```python
from build123d import *

# Parameters (mm, degrees)
BOSS_EXTRUDE1_DEPTH = 0.9


with BuildPart() as part:
    # Sketch1 → Boss-Extrude1 (new body)
    with BuildSketch(Plane(origin=(0, 0, 0), x_dir=(1, 0, 0), z_dir=(0, 1, 0))):
        with BuildLine():
            Line((37, -29.25), (-37, -29.25))
            ThreePointArc((-37, -29.25), (-40.889087297, -27.639087297), (-42.5, -23.75))
            Line((-42.5, -23.75), (-42.5, 23.75))
            ThreePointArc((-42.5, 23.75), (-40.889087297, 27.639087297), (-37, 29.25))
            Line((-37, 29.25), (37, 29.25))
            ThreePointArc((37, 29.25), (40.889087297, 27.639087297), (42.5, 23.75))
            Line((42.5, 23.75), (42.5, -23.75))
            ThreePointArc((42.5, -23.75), (40.889087297, -27.639087297), (37, -29.25))
        make_face()
    extrude(amount=BOSS_EXTRUDE1_DEPTH)

    # Sweep1: sweep along a path in Sketch2
    with BuildLine(Plane(origin=(0, 0.9, 0), x_dir=(1, 0, 0), z_dir=(0, 1, 0))) as sweep1_path:
        Line((34.75, -21.75), (-34.75, -21.75))
        Line((-34.75, -21.75), (-34.75, 21.75))
        Line((-34.75, 21.75), (34.75, 21.75))
        Line((34.75, 21.75), (34.75, -21.75))
    # Sketch3 → Sweep1 (sweep)
    with BuildSketch(Plane.XY):
        with BuildLine():
            Line((-38.25, 0.9), (-31.25, 0.9))
            Line((-31.25, 0.9), (-31.25, 4.4))
            ThreePointArc((-31.25, 4.4), (-34.75, 7.9), (-38.25, 4.4))
            Line((-38.25, 4.4), (-38.25, 0.9))
        make_face()
    sweep(path=sweep1_path.line, transition=Transition.RIGHT)


solid = part.part
```
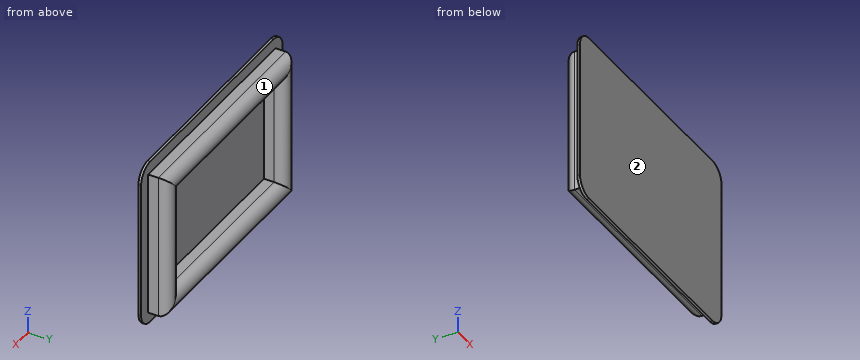
CAD build for the part. Positions are in the model's coordinates, mm. Face numbers are marked on the shaded views. Coordinates: 2 decimals unless noted, no trailing zeros. Order: outer loops, then holes, each group sorted by start corner. A loop starts at its lowest first (then second) coordinate and runs counter-clockwise, first axis right, second up. Notation, with made-up numbers: (-23.75, -7.5) -> (11.25, -7.5) arc R22 ccw to (11.25, 5.5) -> close; hole circle Ø10 at (43.25, -11). An arc over 180 degrees is marked (long way). Use one line per item in the form item = value. Start each with the question number.
1) Band-saw the part on A-A on x = -14.5. Give the cut face in (y, z), then the cut area to 3 significant figures.
2) Band-saw the part on B-B on y = 2.75. Give the cut face in (x, z), then the cut area to 3 significant figures.
3) Band-saw the part on D-D on z = -14. Give the cut face in (x, y), then the cut area to 3 significant figures.
4) Drop flat-ended pins along their axis: pin 1 (17.5 mm diameter, centred on x = -15.5, z = -2, fed in from +Y); pin 2 (3 mm diameter, centred on y = 3.5, z = -6, fed in from -X); pin 3 (1.1 mm diameter, centred on x = -6, y = 2.5, fed in from +Z); pin 4 (4 mm diameter, centred on x = 5.5, y = 2.5, fed in from -Z). Give the stop position or say it passes through.
5) Pull direction Z, two halves, no side cores. Call the marked faces 1 and 2: +Z half, -Z half, draft (parallel to the pull), parting line (faces both ways), or undercut.
6) Band-saw the part on C-C on z = 21.75. Give the cut face in (x, y).
7) Drill centre lines: L1, parallel to X at y = 3, z = 7.5; L2, parallel to Z at x = -27.5, y = 2.5. Where is each one in solid material? Low to high. Write a range as [from, to].
Entries:
q1.outline = (0, -29.25) -> (0.9, -29.25) -> (0.9, -25.25) -> (4.4, -25.25) arc R3.5 ccw to (4.4, -18.25) -> (0.9, -18.25) -> (0.9, 18.25) -> (4.4, 18.25) arc R3.5 ccw to (4.4, 25.25) -> (0.9, 25.25) -> (0.9, 29.25) -> (0, 29.25) -> close
q1.area = 140 mm2
q2.outline = (-38.25, -25.25) -> (38.25, -25.25) -> (38.25, 25.25) -> (-38.25, 25.25) -> close; hole (-31.25, -18.25) -> (31.25, -18.25) -> (31.25, 18.25) -> (-31.25, 18.25) -> close
q2.area = 1,580 mm2
q3.outline = (-42.5, 0) -> (42.5, 0) -> (42.5, 0.9) -> (38.25, 0.9) -> (38.25, 4.4) arc R3.5 ccw to (31.25, 4.4) -> (31.25, 0.9) -> (-31.25, 0.9) -> (-31.25, 4.4) arc R3.5 ccw to (-38.25, 4.4) -> (-38.25, 0.9) -> (-42.5, 0.9) -> close
q3.area = 164 mm2
q4.pin_1 = 0.9
q4.pin_2 = -38.25
q4.pin_3 = 25.25
q4.pin_4 = -29.25
q5.face_1 = undercut
q5.face_2 = draft
q6.outline = (-42.5, 0) -> (42.5, 0) -> (42.5, 0.9) -> (38.25, 0.9) -> (38.25, 4.4) arc R3.5 ccw to (34.75, 7.9) -> (-34.75, 7.9) arc R3.5 ccw to (-38.25, 4.4) -> (-38.25, 0.9) -> (-42.5, 0.9) -> close
q7.L1 = [-38.25, -31.25], [31.25, 38.25]
q7.L2 = [-25.25, -18.25], [18.25, 25.25]
